Here's how the part is built. I have some questions about the finished solid (model axes, mm). Face numbers are marked on the shaded views. A direction names the side the tool comes from. Round coordinates to 2 decimals unless told otherwise and drop trailing zeros. Write each loop counter-clockwise with the first axis right and the second up, starting at its lowest first coordinate (ties: lowest second). Pieces come first, ordered by that corner, then holes. Notation, with made-up numbers: (53, 1) -> (105, 1) arc R25 cw to (105, 38) -> close; hole circle Ø10 at (-17, -20.5). An arc over 180 degrees is marked (long way). Answer in a Markdown table with one row per item. Add a question column.
from build123d import *

# Parameters (mm, degrees)
BOSS_EXTRUDE1_DEPTH         = 5
F_3_3_3_3_DIAMETER_HOLE1_D  = 3.3
FILLET1_RADIUS              = 5
FILLET1_LENGTH              = 4
FILLET2_R                   = 5
F_16_0_177_DIAMETER_HOLE1_D = 4.4958
CUT_EXTRUDE1_DEPTH          = 4


# Read off the part's stored shape, not the designer's step: Cut-Extrude1
with BuildPart() as part:
    # Sketch1 → Boss-Extrude1 (new, symmetric)
    with BuildSketch(Plane.XY):
        Polygon((-16, 0), (16, 0), (16, 4), (2, 4), (2, 20), (-2, 20), (-2, 4), (-16, 4), align=None)
    extrude(amount=BOSS_EXTRUDE1_DEPTH, both=True)

    # Ø3.3 (3.3) Diameter Hole1 (through all)
    with Locations(Plane(origin=(0, 4, 0), x_dir=(1, 0, 0), z_dir=(0, 1, 0))):
        with Locations((-13, 0), (13, 0)):
            Hole(F_3_3_3_3_DIAMETER_HOLE1_D / 2)

    # Fillet1: full round fillet: the end face becomes a half cylinder, R = half its width
    fillet1_face = Plane((0, 20, 0), x_dir=(-1, 0, 0), z_dir=(0, 1, 0))  # on the end face: x along it, z out of the body
    fillet1_slab = fillet1_face.offset(-FILLET1_RADIUS / 2) * Box(FILLET1_LENGTH, 2 * FILLET1_RADIUS, FILLET1_RADIUS, mode=Mode.PRIVATE)  # the body's end, R deep
    fillet1_round = Plane((0, 15, 0), x_dir=(0, 1, 0), z_dir=(-1, 0, 0)) * Cylinder(FILLET1_RADIUS, FILLET1_LENGTH, mode=Mode.PRIVATE)  # its axis R under the face
    add(fillet1_slab - fillet1_round, mode=Mode.SUBTRACT)

    # Fillet2
    fillet2_edges = [part.edges().sort_by_distance(p)[0] for p in [
        (2, 4, 0),
        (-2, 4, 0),
    ]]
    fillet(fillet2_edges, radius=FILLET2_R)

    # #16 (0.177) Diameter Hole1 (through all)
    with Locations(Plane(origin=(2, 0, 0), x_dir=(0, 0, -1), z_dir=(1, 0, 0))):
        with Locations((0, 15)):
            Hole(F_16_0_177_DIAMETER_HOLE1_D / 2)

    # Cut-Extrude1 outline → Cut-Extrude1 (cut)
    with BuildSketch(Plane(origin=(0, 0, 0), x_dir=(1, 0, 0), z_dir=(0, 1, 0))):
        with BuildLine():
            Line((-16, -5), (-11, -5))
            ThreePointArc((-11, -5), (-12.148050297, -4.771638598), (-13.121320344, -4.121320344))
            Line((-13.121320344, -4.121320344), (-15.121320344, -2.121320344))
            ThreePointArc((-15.121320344, -2.121320344), (-15.771638598, -1.148050297), (-16, 0))
            Line((-16, 0), (-16, -5))
        make_face()
        with BuildLine():
            Line((-16, 5), (-16, 0))
            ThreePointArc((-16, 0), (-15.771638598, 1.148050297), (-15.121320344, 2.121320344))
            Line((-15.121320344, 2.121320344), (-13.121320344, 4.121320344))
            ThreePointArc((-13.121320344, 4.121320344), (-12.148050297, 4.771638598), (-11, 5))
            Line((-11, 5), (-16, 5))
        make_face()
    cut_extrude1 = extrude(amount=CUT_EXTRUDE1_DEPTH, mode=Mode.SUBTRACT)

    # Mirror1: Cut-Extrude1 across plane
    add(cut_extrude1.mirror(Plane(origin=(0, 0, 0), x_dir=(0, 0, 1), z_dir=(1, 0, 0))), mode=Mode.SUBTRACT)


solid = part.part
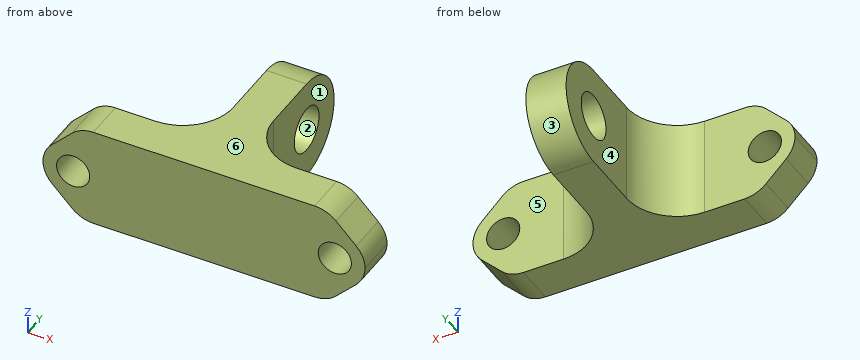
Item 1: For P1, Ø3, axis at y = 16, z = 0.5, coming from the -X side; P2, Ø1, axis at y = 8.5, z = 2, coming from the +X side; P3, Ø1, axis at x = -2, y = 17, coming from the -Z side, each with a flat end and sliding along its axis, tell me the tip position at first contact or that it passes through.
Item 2: I need wall thicknesses on line 1 along Y through (x, z) = (0.8, 0); line 2 along X through (y, z) = (18.75, -2.75); line 3 along Y through (x, z) = (-8.5, -1). Which ranges of each line are inside material? Lowest first, please. Write a range as from..to.
Item 3: If we mould it in two halves opening along Y, with no side actions, what happens to the marked faces 1, 2 and 3? For each: pulls with the +Y half, pulls with the -Y half, needs draft (parallel to the pull), parting line crosses it, or undercut.
Item 4: If we section it at D-D on y = 6: Please give me the cut outline in (x, z).
Item 5: If we section it at A-A on y = 16: Please give me the cut outline in (x, z), then the cut area to 3 significant figures.
Item 6: If we section it at C-C on z = -3.5: Please give me the cut outline in (x, y), then the cut area to 3 significant figures.
Item 7: On a 3-axis mill with a long thin cutter (end or side, diameter ignored), from which of +Z, -Z, +X, -X, +Y, -Y can I reach the whole of each face in a straight line? I mean the marked faces 4, 5 and 6. Say none if no direction works.
Item 8: If we section it at B-B on x = 0: Please give me the cut outline in (y, z), then the cut area to 3 significant figures.
Results list:
| question | item | result |
|---|---|---|
| 1 | P1 | x = -2 |
| 1 | P2 | x = 2.1 |
| 1 | P3 | z = -4.77 |
| 2 | line 1 | 0..12.75, 17.25..20 |
| 2 | line 2 | -2..2 |
| 2 | line 3 | 0..4 |
| 3 | face 1 | needs draft |
| 3 | face 2 | undercut |
| 3 | face 3 | pulls with the +Y half |
| 4 | outline | (-3, -5) -> (3, -5) -> (3, 5) -> (-3, 5) -> close |
| 5 | outline | (-2, -4.9) -> (2, -4.9) -> (2, -2.01) -> (-2, -2.01) -> close; (-2, 2.01) -> (2, 2.01) -> (2, 4.9) -> (-2, 4.9) -> close |
| 5 | area | 23.1 mm² |
| 6 | outline | (-13.74, 0) -> (13.74, 0) -> (13.74, 4) -> (7, 4) arc R5 cw to (2, 9) -> (2, 18.57) -> (-2, 18.57) -> (-2, 9) arc R5 cw to (-7, 4) -> (-13.74, 4) -> close |
| 6 | area | 179 mm² |
| 7 | face 4 | +Z, -Z, -X, +Y |
| 7 | face 5 | +Z, -Z, +X, +Y |
| 7 | face 6 | +Z, +X, -X, +Y, -Y |
| 8 | outline | (0, -5) -> (15, -5) arc R5 ccw to (15, 5) -> (0, 5) -> close; hole circle Ø4.5 at (15, 0) |
| 8 | area | 173 mm² |
